For this review, take the finished solid that the model builds, in its own axes (mm). A direction names the side the tool comes from. Coordinates: 2 decimals unless noted, no trailing zeros. Write each loop counter-clockwise with the first axis right and the second up, starting at its lowest first coordinate (ties: lowest second). Pieces come first, ordered by that corner, then holes. Notation, with made-up numbers: M 80.25,31.5 L 127.25,31.5 A15 ccw 127.25,53.5 Z; hole C -33,3.25 d8. An arc over 180 degrees is marked long. One line per question, with ' | ' between items.
from build123d import *

# Parameters (mm, degrees)
F1_DEPTH  = 3.175
F3_DEPTH  = 2.3622
F5_DEPTH  = 1.5875
F7_DEPTH  = 1.5875
F9_DEPTH  = 2.3876
F11_DEPTH = 2.3876
F12_W     = 1.5875
F12_H     = 7.9375
F13_DEPTH = 25.4


with BuildPart() as f1:
    # F0 (on Front) → F1 (new body)
    with BuildSketch(Plane.XZ):
        with BuildLine():
            Line((-103.2002, -7.9375), (-95.25, -7.9375))
            ThreePointArc((-95.25, -7.9375), (-100.8626600757, -5.6126600757), (-103.1875, 0))
            Line((-103.1875, 0), (-103.2002, 0))
            Line((-103.2002, 0), (-103.2002, -7.9375))
        make_face()
        with BuildLine():
            Line((7.9375, -7.9375), (7.9375, 0))
            ThreePointArc((7.9375, 0), (5.6126600757, -5.6126600757), (0, -7.9375))
            Line((0, -7.9375), (7.9375, -7.9375))
        make_face()
        with BuildLine():
            ThreePointArc((0, -7.9375), (-5.6126600757, -5.6126600757), (-7.9375, 0))
            Line((-7.9375, 0), (-11.1125, 0))
            ThreePointArc((-11.1125, 0), (-13.4373399243, -5.6126600757), (-19.05, -7.9375))
            Line((-19.05, -7.9375), (0, -7.9375))
        make_face()
        with BuildLine():
            Line((-38.1, -7.9375), (-19.05, -7.9375))
            ThreePointArc((-19.05, -7.9375), (-24.6626600757, -5.6126600757), (-26.9875, 0))
            Line((-26.9875, 0), (-30.1625, 0))
            ThreePointArc((-30.1625, 0), (-32.4873399243, -5.6126600757), (-38.1, -7.9375))
        make_face()
        with BuildLine():
            Line((-57.1500000951, -7.9375), (-38.1, -7.9375))
            ThreePointArc((-38.1, -7.9375), (-43.7126600757, -5.6126600757), (-46.0375, 0))
            Line((-46.0375, 0), (-49.2125, 0))
            ThreePointArc((-49.2125, 0), (-51.537339958, -5.6126601093), (-57.1500000951, -7.9375))
        make_face()
        with BuildLine():
            Line((-76.2, -7.9375), (-57.1500000951, -7.9375))
            ThreePointArc((-57.1500000951, -7.9375), (-62.7626601093, -5.612660042), (-65.0875, 0))
            Line((-65.0875, 0), (-68.2625, 0))
            ThreePointArc((-68.2625, 0), (-70.5873399243, -5.6126600757), (-76.2, -7.9375))
        make_face()
        with BuildLine():
            Line((-95.25, -7.9375), (-76.2, -7.9375))
            ThreePointArc((-76.2, -7.9375), (-81.8126600757, -5.6126600757), (-84.1375, 0))
            Line((-84.1375, 0), (-87.3125, 0))
            ThreePointArc((-87.3125, 0), (-89.6373399243, -5.6126600757), (-95.25, -7.9375))
        make_face()
        with BuildLine():
            ThreePointArc((0, -6.35), (-4.4901280605, -4.4901280605), (-6.35, 0))
            Line((-6.35, 0), (-7.9375, 0))
            ThreePointArc((-7.9375, 0), (-5.6126600757, -5.6126600757), (0, -7.9375))
            Line((0, -7.9375), (0, -6.35))
        make_face()
        with BuildLine():
            ThreePointArc((-19.05, -7.9375), (-13.4373399243, -5.6126600757), (-11.1125, 0))
            Line((-11.1125, 0), (-12.7, 0))
            ThreePointArc((-12.7, 0), (-19.05, -6.35), (-25.4, 0))
            Line((-25.4, 0), (-26.9875, 0))
            ThreePointArc((-26.9875, 0), (-24.6626600757, -5.6126600757), (-19.05, -7.9375))
        make_face()
        with BuildLine():
            ThreePointArc((-46.0375, 0), (-43.7126600757, -5.6126600757), (-38.1, -7.9375))
            ThreePointArc((-38.1, -7.9375), (-32.4873399243, -5.6126600757), (-30.1625, 0))
            Line((-30.1625, 0), (-31.75, 0))
            ThreePointArc((-31.75, 0), (-38.1, -6.35), (-44.45, 0))
            Line((-44.45, 0), (-46.0375, 0))
        make_face()
        with BuildLine():
            ThreePointArc((-65.0875, 0), (-62.7626601093, -5.612660042), (-57.1500000951, -7.9375))
            ThreePointArc((-57.1500000951, -7.9375), (-51.537339958, -5.6126601093), (-49.2125, 0))
            Line((-49.2125, 0), (-50.8, 0))
            ThreePointArc((-50.8, 0), (-57.15, -6.35), (-63.5, 0))
            Line((-63.5, 0), (-65.0875, 0))
        make_face()
        with BuildLine():
            ThreePointArc((-84.1375, 0), (-81.8126600757, -5.6126600757), (-76.2, -7.9375))
            ThreePointArc((-76.2, -7.9375), (-70.5873399243, -5.6126600757), (-68.2625, 0))
            Line((-68.2625, 0), (-69.85, 0))
            ThreePointArc((-69.85, 0), (-76.2, -6.35), (-82.55, 0))
            Line((-82.55, 0), (-84.1375, 0))
        make_face()
        with BuildLine():
            Line((-95.25, -6.35), (-95.25, -7.9375))
            ThreePointArc((-95.25, -7.9375), (-89.6373399243, -5.6126600757), (-87.3125, 0))
            Line((-87.3125, 0), (-88.9, 0))
            ThreePointArc((-88.9, 0), (-90.7598719395, -4.4901280605), (-95.25, -6.35))
        make_face()
        with BuildLine():
            ThreePointArc((-103.1875, 0), (-100.8626600757, -5.6126600757), (-95.25, -7.9375))
            Line((-95.25, -7.9375), (-95.25, -6.35))
            ThreePointArc((-95.25, -6.35), (-99.7401280605, -4.4901280605), (-101.6, 0))
            Line((-101.6, 0), (-103.1875, 0))
        make_face()
        with BuildLine():
            Line((7.9375, 0), (6.35, 0))
            ThreePointArc((6.35, 0), (4.4901280605, -4.4901280605), (0, -6.35))
            Line((0, -6.35), (0, -7.9375))
            ThreePointArc((0, -7.9375), (5.6126600757, -5.6126600757), (7.9375, 0))
        make_face()
        with BuildLine():
            ThreePointArc((-82.55, 0), (-76.2, -6.35), (-69.85, 0))
            Line((-69.85, 0), (-70.64375, 0))
            ThreePointArc((-70.64375, 0), (-76.2, -5.55625), (-81.75625, 0))
            Line((-81.75625, 0), (-82.55, 0))
        make_face()
        with BuildLine():
            ThreePointArc((-63.5, 0), (-57.15, -6.35), (-50.8, 0))
            Line((-50.8, 0), (-51.59375, 0))
            ThreePointArc((-51.59375, 0), (-57.15, -5.55625), (-62.70625, 0))
            Line((-62.70625, 0), (-63.5, 0))
        make_face()
        with BuildLine():
            ThreePointArc((-44.45, 0), (-38.1, -6.35), (-31.75, 0))
            Line((-31.75, 0), (-32.54375, 0))
            ThreePointArc((-32.54375, 0), (-38.1, -5.55625), (-43.65625, 0))
            Line((-43.65625, 0), (-44.45, 0))
        make_face()
        with BuildLine():
            ThreePointArc((-25.4, 0), (-19.05, -6.35), (-12.7, 0))
            Line((-12.7, 0), (-13.49375, 0))
            ThreePointArc((-13.49375, 0), (-19.05, -5.55625), (-24.60625, 0))
            Line((-24.60625, 0), (-25.4, 0))
        make_face()
        with BuildLine():
            ThreePointArc((0, -5.55625), (-3.928862053, -3.928862053), (-5.55625, 0))
            Line((-5.55625, 0), (-6.35, 0))
            ThreePointArc((-6.35, 0), (-4.4901280605, -4.4901280605), (0, -6.35))
            Line((0, -6.35), (0, -5.55625))
        make_face()
        with BuildLine():
            Line((6.35, 0), (5.55625, 0))
            ThreePointArc((5.55625, 0), (3.928862053, -3.928862053), (0, -5.55625))
            Line((0, -5.55625), (0, -6.35))
            ThreePointArc((0, -6.35), (4.4901280605, -4.4901280605), (6.35, 0))
        make_face()
        with BuildLine():
            Line((-95.25, -5.55625), (-95.25, -6.35))
            ThreePointArc((-95.25, -6.35), (-90.7598719395, -4.4901280605), (-88.9, 0))
            Line((-88.9, 0), (-89.69375, 0))
            ThreePointArc((-89.69375, 0), (-91.321137947, -3.928862053), (-95.25, -5.55625))
        make_face()
        with BuildLine():
            ThreePointArc((-101.6, 0), (-99.7401280605, -4.4901280605), (-95.25, -6.35))
            Line((-95.25, -6.35), (-95.25, -5.55625))
            ThreePointArc((-95.25, -5.55625), (-99.178862053, -3.928862053), (-100.80625, 0))
            Line((-100.80625, 0), (-101.6, 0))
        make_face()
    extrude(amount=F1_DEPTH)

    # F2 (on face) → F3 (cut)
    with BuildSketch(Plane.XZ.offset(3.175)):
        with BuildLine():
            ThreePointArc((-101.6, 0), (-95.25, -6.35), (-88.9, 0))
            ThreePointArc((-88.9, 0), (-95.25, 6.35), (-101.6, 0))
        make_face()
        with BuildLine():
            ThreePointArc((-82.55, 0), (-76.2, -6.35), (-69.85, 0))
            ThreePointArc((-69.85, 0), (-76.2, 6.35), (-82.55, 0))
        make_face()
        with BuildLine():
            ThreePointArc((-63.5, 0), (-57.15, -6.35), (-50.8, 0))
            ThreePointArc((-50.8, 0), (-57.15, 6.35), (-63.5, 0))
        make_face()
        with BuildLine():
            ThreePointArc((-44.45, 0), (-38.1, -6.35), (-31.75, 0))
            ThreePointArc((-31.75, 0), (-38.1, 6.35), (-44.45, 0))
        make_face()
        with BuildLine():
            ThreePointArc((-25.4, 0), (-19.05, -6.35), (-12.7, 0))
            ThreePointArc((-12.7, 0), (-19.05, 6.35), (-25.4, 0))
        make_face()
        with BuildLine():
            ThreePointArc((-6.35, 0), (0, -6.35), (6.35, 0))
            ThreePointArc((6.35, 0), (0, 6.35), (-6.35, 0))
        make_face()
    extrude(amount=-F3_DEPTH, mode=Mode.SUBTRACT)

    # F4 (on face) → F5 (join)
    with BuildSketch(Plane.YZ.offset(7.9375)):
        Polygon((-2.38125, 0), (-3.175, 0), (-3.175, -7.9375), (0, -7.9375), (0, 0), (-0.79375, 0), (-0.79375, -3.175), (-0.79375, -4.7625), (-2.38125, -4.7625), (-2.38125, -3.175), align=None)
    extrude(amount=F5_DEPTH)

    # F6 (on face) → F7 (join)
    with BuildSketch(Plane(origin=(-103.2002, 0, 0), x_dir=(0, -1, 0), z_dir=(-1, 0, 0))):
        Polygon((0.79375, 0), (0, 0), (0, -7.9375), (3.175, -7.9375), (3.175, 0), (2.38125, 0), (2.38125, -3.175), (2.38125, -4.7625), (0.79375, -4.7625), (0.79375, -3.175), align=None)
    extrude(amount=F7_DEPTH)

    # F8 (on face) → F9 (join)
    with BuildSketch(Plane(origin=(0, 0, 0), x_dir=(-1, 0, 0), z_dir=(0, 1, 0))):
        Polygon((-7.9375, -3.175), (-7.9375, 0), (-9.525, -3.175), align=None)
    extrude(amount=-F9_DEPTH)

    # F10 (on face) → F11 (join)
    with BuildSketch(Plane(origin=(0, 0, 0), x_dir=(-1, 0, 0), z_dir=(0, 1, 0))):
        Polygon((104.7877, -3.175), (103.99395, 0), (103.99395, -3.175), align=None)
    extrude(amount=-F11_DEPTH)

    # F12 (on face) → F13 (cut)
    with BuildSketch(Plane.XZ.offset(3.175)):
        with Locations((8.73125, -3.96875)):
            Rectangle(F12_W, F12_H)
        with Locations((-103.99395, -3.96875)):
            Rectangle(F12_W, F12_H)
    extrude(amount=-F13_DEPTH, mode=Mode.SUBTRACT)


solid = f1.part
1) The part is to be moulded in two halves that separate along Z. For faces 1 (the flat face through (-47, -2, -7.938)), 2 (the flat face through (-103.2, -2, -4)), 3 (the cylindrical face through (-18.928, -0.401, -5.555)), say which applies: +Z half, -Z half, draft (parallel to the pull), parting line (faces both ways), or undercut.
Responses:
face 1: -Z half | face 2: draft | face 3: +Z half
2) Machinability: for faces 4 (the flat face through (-67, -2, 0)), 5 (the flat face through (1, -0.813, -6)), which of the approach directions +Z, -Z, +X, -X, +Y, -Y give a long, thin tool a straight path to every point of the face, cutting with its end or side? Answer none if there is none.
Responses:
face 4: +Z, +X, -X, +Y, -Y | face 5: +Z, -Y
3) Insertion check: pin 1 Ø3 at (x, z) = (-94, -4) entering from -Y. The pin has a flat end and moves straight along its axis. Give the tip position at first contact, or say it passes through.
Responses:
pin 1: y = -0.81
4) To check wall thickness, follow line 1 along Z through (x, y) = (-19, -2.85); line 2 along Z through (x, y) = (-90, -2.05). State the ranges of each line that lie inside material, in increasing order. Write a range as [from, to].
Responses:
line 1: [-7.94, -6.35] | line 2: [-7.94, -3.57]
5) We need section C-C on z = -3.25. State how many separate pieces and enclosed holes the cut face has, then the cut area to 3 significant figures.
Responses:
separate pieces: 7 | enclosed holes: 0 | area: 154 mm^2
6) We need section A-A on y = -2.65. State the section outline as (x, z) points, then the cut area to 3 significant figures.
Responses:
outline: M -103.2,-7.94 L 7.94,-7.94 L 7.94,0 L 6.35,0 A6.35 cw -6.35,0 L -12.7,0 A6.35 cw -25.4,0 L -31.75,0 A6.35 cw -44.45,0 L -50.8,0 A6.35 cw -63.5,0 L -69.85,0 A6.35 cw -82.55,0 L -88.9,0 A6.35 cw -101.6,0 L -103.2,0 Z | area: 502 mm^2
